Print and shaded views of the part. All mm, measured from the part's lowest x, y and z. A direction names the side the tool comes from. Round coordinates to 2 decimals unless told otherwise and drop trailing zeros. Loops run counter-clockwise (first coordinate to the right, second up) from the corner with the lowest first, then second, coordinate; pieces in that order, holes last. Notation, with made-up numbers: (70.25, 49.5) -> (74.25, 49.5) arc R14 ccw to (74.25, 68.5) -> close; hole circle Ø9 at (-11.75, -6). An arc over 180 degrees is marked (long way). Answer as CSV lines item,"result".
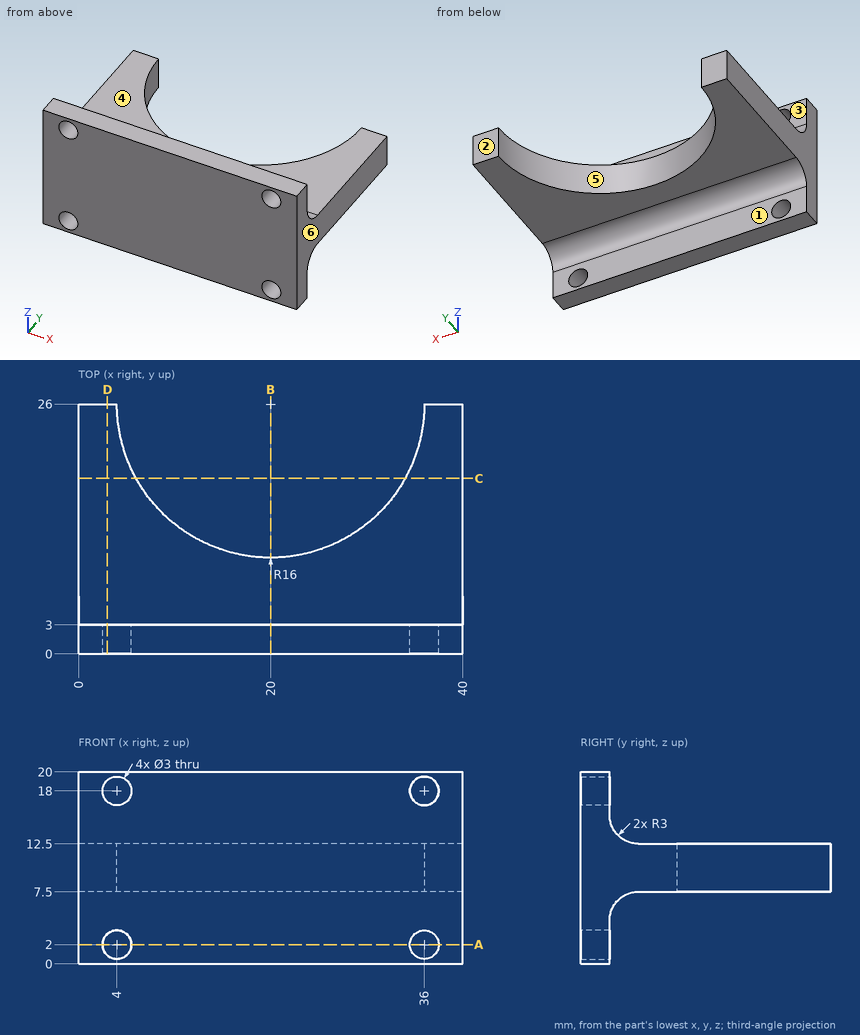
Q1. Probe L1, parallel to X at y = 2.35, z = 18; L2, parallel to Z at x = 4, y = 1; L3, parallel to Y at x = 29.5, z = 16. List the from-to ranges inside material, lowest first. Write a range as [from, to].
Results:
L1,"[0, 2.5], [5.5, 34.5], [37.5, 40]"
L2,"[0, 0.5], [3.5, 16.5], [19.5, 20]"
L3,"[0, 3]"
Q2. Slice it at B-B, the plane x = 20. Give the cut face in (y, z).
Results:
outline,"(0, 0) -> (3, 0) -> (3, 4.5) arc R3 cw to (6, 7.5) -> (10, 7.5) -> (10, 12.5) -> (6, 12.5) arc R3 cw to (3, 15.5) -> (3, 20) -> (0, 20) -> close"
Q3. Tool access for the marked faces 1, 2 and 3: list every direction of +Z, -Z, +X, -X, +Y, -Y with a clear straight run to the whole face (end or side of a thin tool).
Results:
face 1,"-Z, +X, -X, +Y"
face 2,"+Z, -Z, +X, -X, +Y"
face 3,"+Z, +X, -X, +Y"
Q4. Slice it at D-D, the plane x = 3. Give the cut face in (y, z).
Results:
outline,"(0, 0) -> (3, 0) -> (3, 0.88) -> (0, 0.88) -> close; (0, 3.12) -> (3, 3.12) -> (3, 4.5) arc R3 cw to (6, 7.5) -> (26, 7.5) -> (26, 12.5) -> (6, 12.5) arc R3 cw to (3, 15.5) -> (3, 16.88) -> (0, 16.88) -> close; (0, 19.12) -> (3, 19.12) -> (3, 20) -> (0, 20) -> close"
Q5. Slice it at A-A, the plane z = 2. Give the cut face in (x, y).
Results:
outline,"(0, 0) -> (2.5, 0) -> (2.5, 3) -> (0, 3) -> close; (5.5, 0) -> (34.5, 0) -> (34.5, 3) -> (5.5, 3) -> close; (37.5, 0) -> (40, 0) -> (40, 3) -> (37.5, 3) -> close"
Q6. Two-plate mould, pull along X, no slides. Class the marked faces 4, 5 and 6: pulls with the +X half, pulls with the -X half, needs draft (parallel to the pull), parting line crosses it, or undercut.
Results:
face 4,"needs draft"
face 5,"undercut"
face 6,"pulls with the +X half"
Q7. Slice it at C-C, the plane y = 18.25. Give the cut face in (x, z), and give its area (3 significant figures).
Results:
outline,"(0, 7.5) -> (6, 7.5) -> (6, 12.5) -> (0, 12.5) -> close; (34, 7.5) -> (40, 7.5) -> (40, 12.5) -> (34, 12.5) -> close"
area,"60.0 mm2"
Q8. Drop flat-ended pins along their axis: pin 1 Ø1 at (x, z) = (5.5, 14) entering from +Y; pin 2 Ø1.5 at (x, y) = (23.5, 4.5) entering from -Z; pin 3 Ø2 at (x, z) = (11, 17) entering from +Y; pin 4 Ø3 at (y, z) = (20.5, 5) entering from -X. Give the stop position or say it passes through.
Results:
pin 1,"y = 3.76"
pin 2,"z = 6.48"
pin 3,"y = 3"
pin 4,"through"
